```python
from build123d import *

# Parameters (mm, degrees)
F0_W      = 50
F0_H      = 50
F1_DEPTH  = 3
F2_W      = 30
F2_H      = 6
F3_DEPTH  = 40
F4_W      = 30
F4_H      = 6
F5_DEPTH  = 40
F6_R      = 14.99999
F7_R      = 14.99999
F9_D      = 5
F12_D     = 4
F12_DEPTH = 15
F12_TIP   = 1.2017212381


# Not quite as in the source:
# - a fillet or chamfer is up to 0.001 mm smaller than in the source, because OpenCascade refuses the exact size


with BuildPart() as f1:
    # F0 (on Top) → F1 (new body)
    with BuildSketch(Plane.XY):
        with Locations((1.1680303141, 2.4703653681)):
            Rectangle(F0_W, F0_H)
    extrude(amount=F1_DEPTH)

    # F2 (on face) → F3 (join)
    with BuildSketch(Plane.XY.offset(3)):
        with Locations((1.1680303141, -6.0296346319)):
            Rectangle(F2_W, F2_H)
    extrude(amount=F3_DEPTH)

    # F4 (on face) → F5 (join)
    with BuildSketch(Plane.XY.offset(3)):
        with Locations((1.1680303141, 10.4703653681)):
            Rectangle(F4_W, F4_H)
    extrude(amount=F5_DEPTH)

    # F6 (radius 15 in the source; OpenCascade refuses exactly that, so slightly less here)
    f6_edges = [f1.edges().sort_by_distance(p)[0] for p in [
        (-13.83197, -6.029635, 43),
        (16.16803, -6.029635, 43),
    ]]
    fillet(f6_edges, radius=F6_R)

    # F7 (radius 15 in the source; OpenCascade refuses exactly that, so slightly less here)
    f7_edges = [f1.edges().sort_by_distance(p)[0] for p in [
        (16.16803, 10.470365, 43),
        (-13.83197, 10.470365, 43),
    ]]
    fillet(f7_edges, radius=F7_R)

    # F9 (through all)
    with Locations(Plane.XZ.offset(9.0296346319)):
        with Locations((1.1680303141, 37.8934629261)):
            Hole(F9_D / 2)

    # F12
    with Locations(Plane.XY.offset(3)):
        with Locations((-17.8319696859, 21.4703653681), (20.1680303141, 21.4703653681), (20.1680303141, -16.5296346319), (-17.8319696859, -16.5296346319)):
            Hole(F12_D / 2, depth=F12_DEPTH)
            with Locations((0, 0, -(F12_DEPTH + F12_TIP / 2))):  # 118° drill point
                Cone(0, F12_D / 2, F12_TIP, mode=Mode.SUBTRACT)


solid = f1.part
```
Check sheet for the modelled part. Datum: model origin and axes. Units: mm. A direction names the side the tool comes from. Round coordinates to 2 decimals unless told otherwise and drop trailing zeros. Write each loop counter-clockwise with the first axis right and the second up, starting at its lowest first coordinate (ties: lowest second). Pieces come first, ordered by that corner, then holes. Notation, with made-up numbers: M -8,1 L 46,1 A31 cw 46,34 Z; hole C 83.5,30 d4. An arc over 180 degrees is marked long. Write item = value, one per line. Start each with the question number.
1. Section check D-D, the plane z = 37. Record the cut outline in (x, y).
2. Scan lines: line 1 (Y direction, x = 1, z = 30.5); line 2 (Z direction, x = -18, y = 0.5); line 3 (X direction, y = 9.5, z = 33). Record each from-to range of solid material in increasing order. Write a range as [from, to].
3. Tool access check on faces 1 (the flat face through (1, 13.47, 23)), 2 (the flat face through (16.168, -6, 15)), 3 (the flat face through (-13.832, -6, 15)), 4 (the flat face through (1, -3.03, 23)). Record the directions out of +Z, -Z, +X, -X, +Y, -Y that give a thin tool (end or side, any length) a straight path to the whole face; none if there is none.
4. Release check for a two-part mould opening along X. For faces 5 (the cylindrical face through (-9.555, -5.988, 38.489)), 6 (the cylindrical face through (-19.74, -15.93, 1.48)), 7 (the flat face through (26.168, 2, 1)) record: pulls with the +X half, pulls with the -X half, needs draft (parallel to the pull), parting line crosses it, or undercut.
5. Section check A-A, the plane z = 5. Record the cut outline in (x, y).
6. Section check C-C, the plane x = 6. Record the cut outline in (y, z), then the cut area to 3 significant figures.
7. Gauge pin test, flat ends, axial feed: pin 1 (6.5 mm diameter, centred on x = 20.17, y = 21.47, fed in from +Z); pin 2 (6.5 mm diameter, centred on y = -7, z = 15, fed in from -X); pin 3 (5 mm diameter, centred on y = -6, z = 20.5, fed in from +X). Record the tip position at first contact, or that the pin passes through.
Results found:
q1.outline = M -10.83,-9.03 L -1.17,-9.03 L -1.17,-3.03 L -10.83,-3.03 Z; M -10.83,7.47 L -1.17,7.47 L -1.17,13.47 L -10.83,13.47 Z; M 3.5,-9.03 L 13.17,-9.03 L 13.17,-3.03 L 3.5,-3.03 Z; M 3.5,7.47 L 13.17,7.47 L 13.17,13.47 L 3.5,13.47 Z
q2.line_1 = [-9.03, -3.03], [7.47, 13.47]
q2.line_2 = [0, 3]
q2.line_3 = [-12.97, 15.31]
q3.face_1 = +Z, +X, -X, +Y
q3.face_2 = +Z, +X, +Y, -Y
q3.face_3 = +Z, -X, +Y, -Y
q3.face_4 = +Z, +X, -X
q4.face_5 = pulls with the -X half
q4.face_6 = undercut
q4.face_7 = pulls with the +X half
q5.outline = M -13.83,-9.03 L 16.17,-9.03 L 16.17,-3.03 L -13.83,-3.03 Z; M -13.83,7.47 L 16.17,7.47 L 16.17,13.47 L -13.83,13.47 Z
q6.outline = M -22.53,0 L 27.47,0 L 27.47,3 L 13.47,3 L 13.47,42.2 L 7.47,42.2 L 7.47,3 L -3.03,3 L -3.03,42.2 L -9.03,42.2 L -9.03,3 L -22.53,3 Z
q6.area = 620 mm^2
q7.pin_1 = 3
q7.pin_2 = -13.83
q7.pin_3 = 16.17
